Here's the drawing with two shaded views (mm, measured from the low corner). I have some questions. A direction names the side the tool comes from. Give positions to 0.01 mm unless a question says otherwise; leave off trailing zeros. Loops run counter-clockwise (first coordinate to the right, second up) from the corner with the lowest first, then second, coordinate; pieces in that order, holes last. Notation, with made-up numbers: M 50,-28.75 L 65,-28.75 A23 ccw 65,-17.75 Z; hole C -15,75 d7. An arc over 180 degrees is marked long. Use CSV: the item, a comma, the result in double quotes.
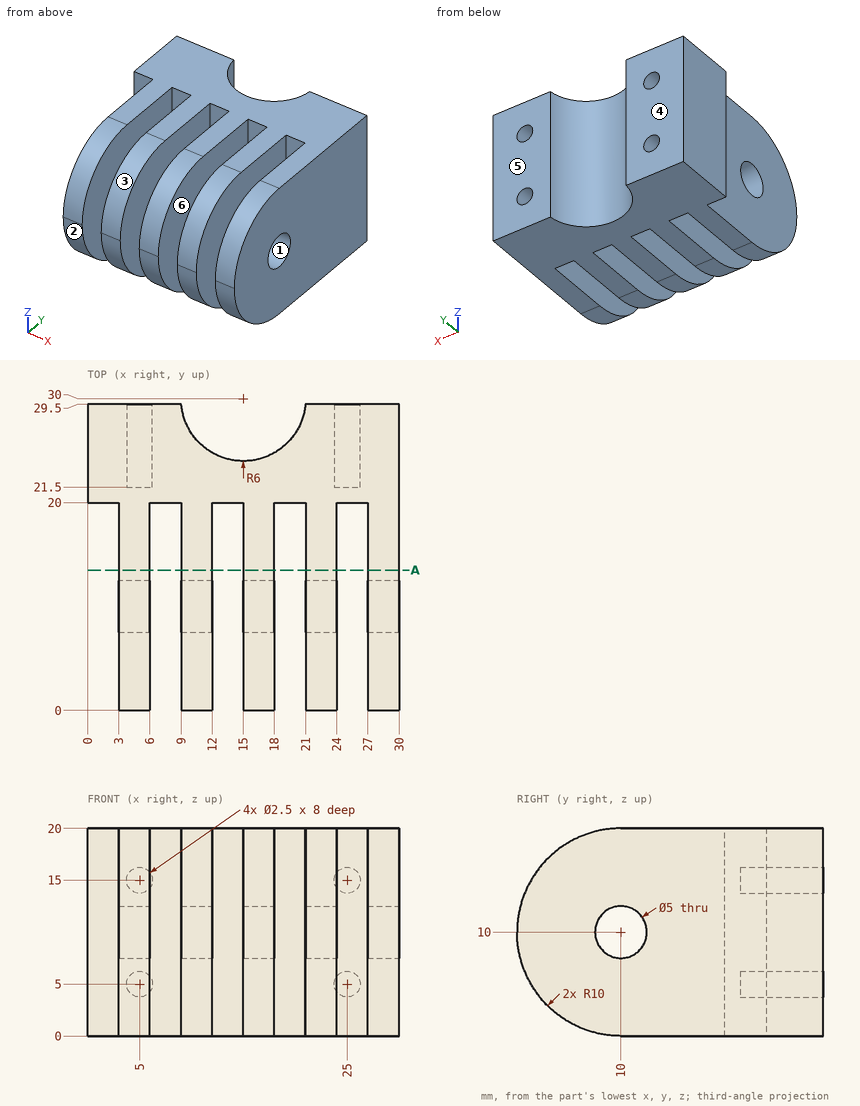
1. Which directions (+Z, -Z, +X, -X, +Y, -Y) give clear straight access to the entire face, cutting with the end or side of a thin tool? Please do the marked faces 5 and 6.
Outcome:
face 5,"+Z, -Z, +X, -X, +Y"
face 6,"+Z, -Z, -Y"
2. I'm going to push flat-ended pins straight in: pin 1 Ø5 at (x, z) = (13, 9) entering from +Y; pin 2 Ø3 at (y, z) = (12, 3) entering from -X; pin 3 Ø0.7 at (x, z) = (5.5, 15) entering from +Y; pin 4 Ø4 at (y, z) = (10, 10) entering from -X. Where does each tip first touch, or does it pass through?
Outcome:
pin 1,"y = 26.03"
pin 2,"x = 3"
pin 3,"y = 21.5"
pin 4,"through"
3. Please list where these lines run through material, in increasing order: line 1 (X direction, y = 15.5, z = 19); line 2 (Z direction, x = 11.1, y = 10); line 3 (X direction, y = 23, z = 14.25).
Outcome:
line 1,"3 to 6, 9 to 12, 15 to 18, 21 to 24, 27 to 30"
line 2,"0 to 7.5, 12.5 to 20"
line 3,"0 to 4, 6 to 24, 26 to 30"
4. I want a section at A-A, the plane y = 13.5. List the corners of the cut face in (x, z) for me, then the cut area to 3 significant figures.
Outcome:
outline,"M 3,0 L 6,0 L 6,20 L 3,20 Z; M 9,0 L 12,0 L 12,20 L 9,20 Z; M 15,0 L 18,0 L 18,20 L 15,20 Z; M 21,0 L 24,0 L 24,20 L 21,20 Z; M 27,0 L 30,0 L 30,20 L 27,20 Z"
area,"300 mm2"
5. If we mould it in two halves opening along Z, with no side actions, what happens to the marked faces 1, 2, 3 and 4? For each: +Z half, -Z half, draft (parallel to the pull), parting line (faces both ways), or undercut.
Outcome:
face 1,"undercut"
face 2,"-Z half"
face 3,"+Z half"
face 4,"draft"
